from build123d import *

# Parameters (mm, degrees)
F0_R     = 3.15
F1_DEPTH = 28
F2_R     = 2.5
F3_DEPTH = 8


# Not quite as in the source:
# - a pattern or mirror of a feature is missing from the dataset's text; its kind, count and spacing are read off the source's solid


with BuildPart() as f1:
    # F0 (on Front) → F1 (new body, symmetric)
    with BuildSketch(Plane.XZ):
        Circle(F0_R)
    extrude(amount=F1_DEPTH, both=True)

    # F2 (on face) → F3 (join)
    with BuildSketch(Plane.XZ.offset(28)):
        Circle(F2_R)
    f3 = extrude(amount=F3_DEPTH)

    # F3_copies: F3 across plane
    add(f3.mirror(Plane.ZX))


solid = f1.part
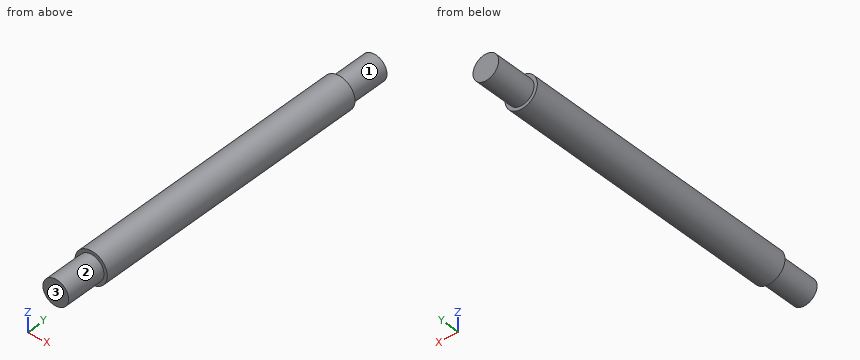
The listing builds one solid part. Answer for the finished solid, in the listing's coordinates (mm). Face numbers are marked on the shaded views. A direction names the side the tool comes from. Coordinates: 2 decimals unless noted, no trailing zeros. Write each loop counter-clockwise with the first axis right and the second up, starting at its lowest first coordinate (ties: lowest second). Pieces come first, ordered by that corner, then holes. Notation, with made-up numbers: M 9,-8.5 L 64,-8.5 A29 ccw 64,26.5 Z; hole C 21.5,-6.5 d1. An arc over 180 degrees is marked long. Put each result on its own line as item: value. Start each with the question number.
1. Consider line 1 (Y direction, x = 2.75, z = -1.25); line 2 (Z direction, x = 0.25, y = -24.5). Determine where each line is inside the solid, lowest interval first. Write a range as from..to.
2. Which of the six approach directions +Z, -Z, +X, -X, +Y, -Y give full straight-line access (tool end or side, diameter ignored) to the marked faces 1, 2 and 3?
3. A cutting plane is placed at A-A on z = 0. Write down the section's boundary in (x, y), then the cut area to 3 significant figures.
4. A cutting plane is placed at C-C on y = -21.5. Write down the section's boundary in (x, z).
5. A cutting plane is placed at B-B on x = 0. Write down the section's boundary in (y, z), then the cut area to 3 significant figures.
6. Flat-ended cylindrical pins translate along their axes: P1, Ø3, axis at x = 2, y = 6, coming from the +Z side; P2, Ø1.5, axis at x = 1.5, y = -16.5, coming from the -Z side. Find the tip coordinate at first contact, or state that the pin passes through.
Resolved:
1. line 1: y = -28..28
1. line 2: z = -3.14..3.14
2. face 1: +Y
2. face 2: -Y
2. face 3: +Z, -Z, +X, -X, -Y
3. outline: M -3.15,-28 L -2.5,-28 L -2.5,-36 L 2.5,-36 L 2.5,-28 L 3.15,-28 L 3.15,28 L 2.5,28 L 2.5,36 L -2.5,36 L -2.5,28 L -3.15,28 Z
3. area: 433 mm2
4. outline: C 0,0 d6.3
5. outline: M -36,-2.5 L -28,-2.5 L -28,-3.15 L 28,-3.15 L 28,-2.5 L 36,-2.5 L 36,2.5 L 28,2.5 L 28,3.15 L -28,3.15 L -28,2.5 L -36,2.5 Z
5. area: 433 mm2
6. P1: stops at z = 3.11
6. P2: stops at z = -3.06
